Input: dimensioned drawing with shaded views. Units: mm. Origin: part minimum x, y, z. Round coordinates to 2 decimals unless told otherwise and drop trailing zeros. Write each loop counter-clockwise with the first axis right and the second up, starting at its lowest first coordinate (ties: lowest second). Pieces come first, ordered by that corner, then holes. Notation, with made-up numbers: M -10,-14.5 L 29,-14.5 A20 cw 29,-4.5 Z; hole C 4.25,51.25 d7. An arc over 180 degrees is marked long. Answer in a Markdown table with one row per item. Add a question column.
Item 1: Cut plane A-A on z = 56. Return loops of the section in (x, y), and give its area (3 significant figures).
Item 2: Cut plane D-D on z = 10. Return loops of the section in (x, y), and give its area (3 significant figures).
Item 3: Material intervals for probe 1 along Y at (x, z) = (1.05, 56); probe 2 along Y at (x, z) = (2.6, 72.75) (1 decimal); probe 3 along Z at (x, y) = (1.95, 67), sorted ascending.
Item 4: Contact query for flat-ended pins moving along their axis: pin 1 (3.5 mm diameter, centred on y = 65, z = 93, fed in from +X); pin 2 (1.5 mm diameter, centred on x = 1, z = 74.5, fed in from +Y); pin 3 (1 mm diameter, centred on x = 0.5, y = 82, fed in from +Z). Output: stop coordinate, or through.
Item 5: Cut plane C-C on y = 33. Return loops of the section in (x, z).
Item 6: Cut plane B-B on x = 2.2. Give the number of separate pieces and of enclosed holes in the cut face, and give its area (3 significant figures).
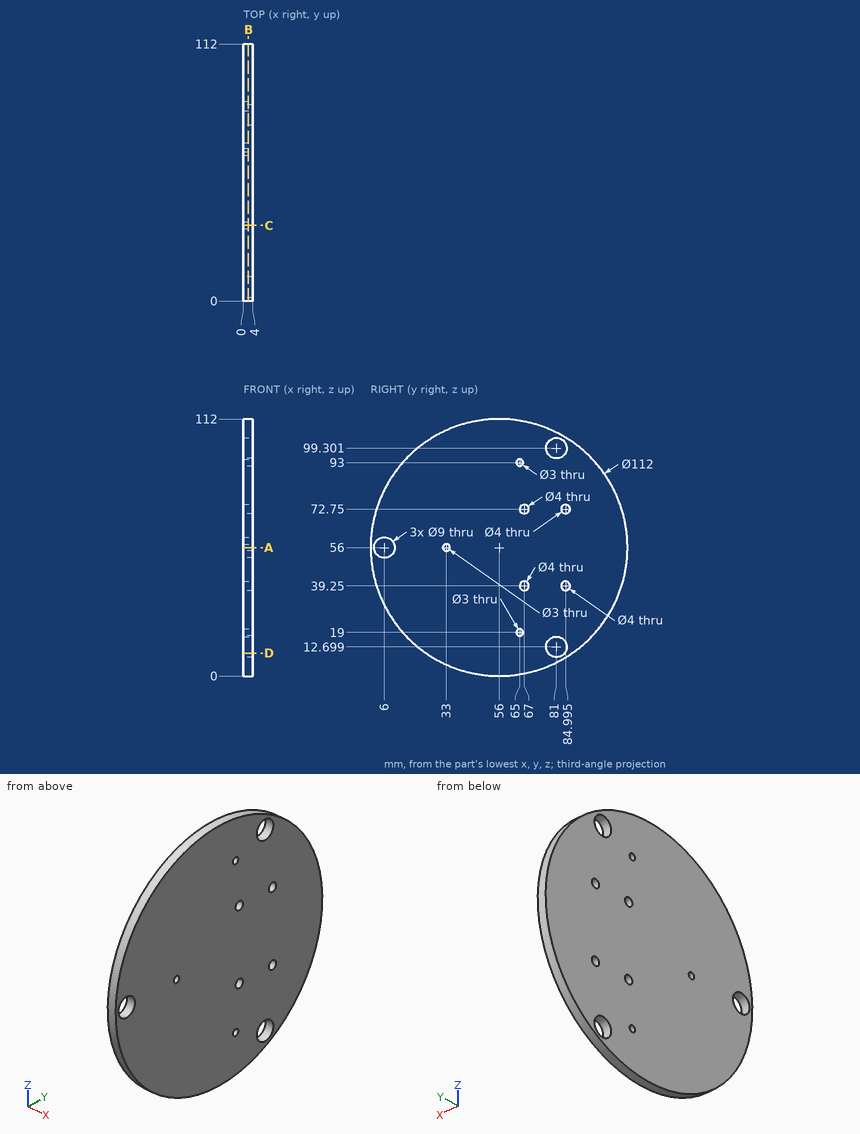
Results below:
| question | item | result |
|---|---|---|
| 1 | outline | M 0,0 L 4,0 L 4,1.5 L 0,1.5 Z; M 0,10.5 L 4,10.5 L 4,31.5 L 0,31.5 Z; M 0,34.5 L 4,34.5 L 4,112 L 0,112 Z |
| 1 | area | 400 mm2 |
| 2 | outline | M 0,24.06 L 4,24.06 L 4,77.4 L 0,77.4 Z; M 0,84.6 L 4,84.6 L 4,87.94 L 0,87.94 Z |
| 2 | area | 227 mm2 |
| 3 | probe 1 | 0 to 1.5, 10.5 to 31.5, 34.5 to 112 |
| 3 | probe 2 | 2.6 to 65, 69 to 83, 87 to 109.4 |
| 3 | probe 3 | 1.09 to 37.25, 41.25 to 70.75, 74.75 to 110.91 |
| 4 | pin 1 | x = 4 |
| 4 | pin 2 | y = 109.11 |
| 4 | pin 3 | z = 105.86 |
| 5 | outline | M 0,4.94 L 4,4.94 L 4,54.5 L 0,54.5 Z; M 0,57.5 L 4,57.5 L 4,107.06 L 0,107.06 Z |
| 6 | separate pieces | 1 |
| 6 | enclosed holes | 10 |
| 6 | area | 9,590 mm2 |
